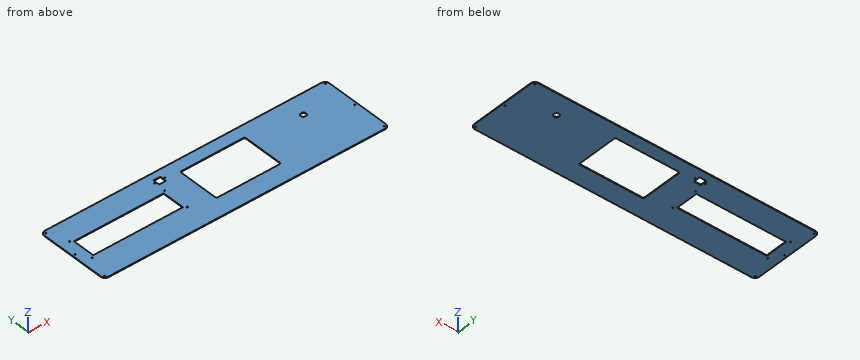
```python
from build123d import *

# Parameters (mm, degrees)
F0_W     = 1371.6
F0_H     = 355.6
F0_R     = 2.54
F0_R_2   = 2.413
F0_W_2   = 431.8
F0_H_2   = 107.95
F0_R_3   = 2.5
F0_W_3   = 33.02
F0_H_3   = 31.75
F0_R_4   = 12.7
F1_DEPTH = 3.175
F2_R     = 20.32


with BuildPart() as f1:
    # F0 (on Top) → F1 (new body)
    with BuildSketch(Plane.XY):
        with Locations((685.8, 177.8)):
            Rectangle(F0_W, F0_H)
        with Locations((12.7, 12.7)):
            Circle(F0_R, mode=Mode.SUBTRACT)
        with Locations((47.227706, 121.980773)):
            Circle(F0_R_2, mode=Mode.SUBTRACT)
        with Locations((504.427706, 121.980773)):
            Circle(F0_R_2, mode=Mode.SUBTRACT)
        with Locations((1358.9, 12.7)):
            Circle(F0_R, mode=Mode.SUBTRACT)
        with Locations((12.7, 177.8)):
            Circle(F0_R, mode=Mode.SUBTRACT)
        with Locations((275.827706, 185.480773)):
            Rectangle(F0_W_2, F0_H_2, mode=Mode.SUBTRACT)
        with Locations((47.227706, 248.980773)):
            Circle(F0_R_2, mode=Mode.SUBTRACT)
        with Locations((504.427706, 248.980773)):
            Circle(F0_R_2, mode=Mode.SUBTRACT)
        with Locations((12.7, 342.9)):
            Circle(F0_R, mode=Mode.SUBTRACT)
        with Locations((505.246378, 305.110961)):
            Circle(F0_R_3, mode=Mode.SUBTRACT)
        with Locations((529.376378, 305.110961)):
            Rectangle(F0_W_3, F0_H_3, mode=Mode.SUBTRACT)
        with Locations((553.506378, 305.110961)):
            Circle(F0_R_3, mode=Mode.SUBTRACT)
        with BuildLine():
            ThreePointArc((619.385123, 289.537351), (621.244995, 294.027479), (625.735123, 295.887351))
            Line((625.735123, 295.887351), (924.185123, 295.887351))
            ThreePointArc((924.185123, 295.887351), (928.675251, 294.027479), (930.535123, 289.537351))
            Line((930.535123, 289.537351), (930.535123, 99.037351))
            ThreePointArc((930.535123, 99.037351), (928.675251, 94.547223), (924.185123, 92.687351))
            Line((924.185123, 92.687351), (625.735123, 92.687351))
            ThreePointArc((625.735123, 92.687351), (621.244995, 94.547223), (619.385123, 99.037351))
            Line((619.385123, 99.037351), (619.385123, 289.537351))
        make_face(mode=Mode.SUBTRACT)
        with Locations((1358.9, 177.8)):
            Circle(F0_R, mode=Mode.SUBTRACT)
        with Locations((1179.455161, 256.812692)):
            Circle(F0_R_4, mode=Mode.SUBTRACT)
        with Locations((1358.9, 342.9)):
            Circle(F0_R, mode=Mode.SUBTRACT)
    extrude(amount=F1_DEPTH)

    # F2
    f2_edges = [f1.edges().sort_by_distance(p)[0] for p in [
        (0, 355.6, 1.5875),
        (0, 0, 1.5875),
        (1371.6, 0, 1.5875),
        (1371.6, 355.6, 1.5875),
    ]]
    fillet(f2_edges, radius=F2_R)


solid = f1.part
```
Input: part model. Units: mm. Frame: model coordinates. Coordinates: 2 decimals unless noted, no trailing zeros. Loops run counter-clockwise (first coordinate to the right, second up) from the corner with the lowest first, then second, coordinate; pieces in that order, holes last. Notation, with made-up numbers: M 39,23.25 L 93,23.25 A25 ccw 93,40.25 Z; hole C 55.25,60 d1. An arc over 180 degrees is marked long. Answer in a Markdown table with one row per item.
1. Section C-C, the plane z = 1. Count the separate pieces of the cut face and the enclosed holes in it, then the cut area to 3 significant figures.
Response:
| item | result |
|---|---|
| separate pieces | 1 |
| enclosed holes | 16 |
| area | 376,000 mm2 |
2. Section A-A, the plane x = 451.5. Output: boundary loops of the cut face in (y, z) (3 decimals), then the cut area to 3 significant figures.
Response:
| item | result |
|---|---|
| outline | M 0,0 L 131.506,0 L 131.506,3.175 L 0,3.175 Z; M 239.456,0 L 355.6,0 L 355.6,3.175 L 239.456,3.175 Z |
| area | 786 mm2 |
3. Material intervals for line 1 (X direction, y = 177.8, z = 0.85); line 2 (X direction, y = 225.5, z = 0.5); line 3 (Y direction, x = 347.5, z = 0.45), sorted ascending.
Response:
| item | result |
|---|---|
| line 1 | x = 0 to 10.16, 15.24 to 59.93, 491.73 to 619.39, 930.54 to 1356.36, 1361.44 to 1371.6 |
| line 2 | x = 0 to 59.93, 491.73 to 619.39, 930.54 to 1371.6 |
| line 3 | y = 0 to 131.51, 239.46 to 355.6 |
4. First-contact query: pin 1 (4 mm diameter, centred on x = 1358.9, y = 342.9, fed in from +Z). Flat tip, straight axial feed; report the tip coordinate or a pass-through.
Response:
| item | result |
|---|---|
| pin 1 | passes through |
5. Section B-B, the plane y = 210. Output: boundary loops of the cut face in (x, z) (3 decimals), then the cut area to 3 significant figures.
Response:
| item | result |
|---|---|
| outline | M 0,0 L 59.928,0 L 59.928,3.175 L 0,3.175 Z; M 491.728,0 L 619.385,0 L 619.385,3.175 L 491.728,3.175 Z; M 930.535,0 L 1371.6,0 L 1371.6,3.175 L 930.535,3.175 Z |
| area | 2,000 mm2 |
